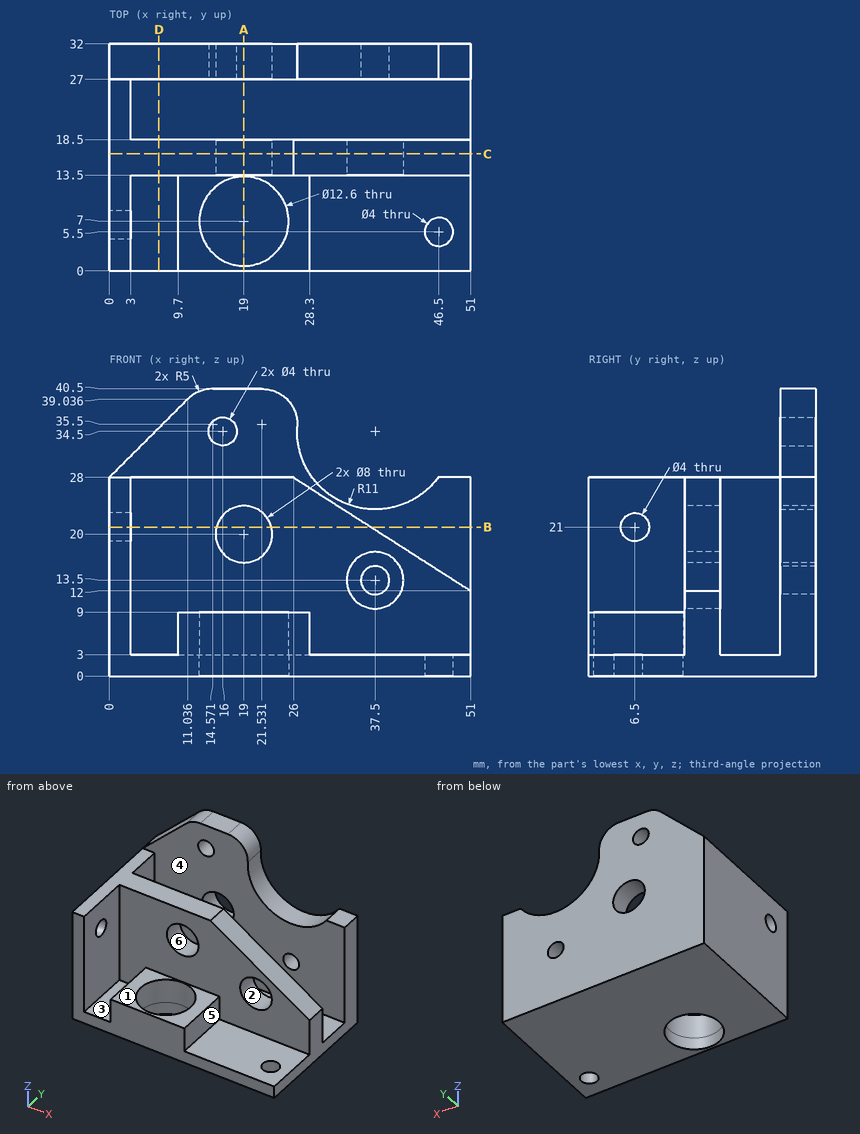
Part print with two shaded views. Sizes in mm from the minimum x, y, z corner. A direction names the side the tool comes from. Round coordinates to 2 decimals unless told otherwise and drop trailing zeros. Write each loop counter-clockwise with the first axis right and the second up, starting at its lowest first coordinate (ties: lowest second). Pieces come first, ordered by that corner, then holes. Notation, with made-up numbers: (-19.75, 60) - (28.25, 60) arc R34 ccw to (28.25, 90) - close; hole circle Ø7 at (-22.5, 8.25). An arc over 180 degrees is marked (long way). Use CSV: the item, a comma, the result in double quotes.
Item 1: Slice it at A-A, the plane x = 19. Write the cut outline in (y, z).
Results list:
outline,"(0, 0) - (0.7, 0) - (0.7, 9) - (0, 9) - close; (13.3, 0) - (32, 0) - (32, 16) - (27, 16) - (27, 3) - (18.5, 3) - (18.5, 16) - (13.5, 16) - (13.5, 9) - (13.3, 9) - close; (13.5, 24) - (18.5, 24) - (18.5, 28) - (13.5, 28) - close; (27, 24) - (32, 24) - (32, 40.5) - (27, 40.5) - close"
Item 2: Flat gauge pins, fed straight in: P1, Ø3.5, axis at y = 6.5, z = 21, coming from the -X side; P2, Ø4, axis at y = 22, z = 18, coming from the +X side; P3, Ø3, axis at x = 16.5, y = 21, coming from the +Z side; P4, Ø1.8, axis at y = 9, z = 5, coming from the +X side. Where does each tip first touch, or does it go through?
Results list:
P1,"passes through"
P2,"stops at x = 3"
P3,"stops at z = 3"
P4,"stops at x = 28.3"
Item 3: Slice it at B-B, the plane z = 21. Write the cut outline in (x, y), then the cut area to 3 significant figures.
Results list:
outline,"(0, 0) - (3, 0) - (3, 4.5) - (0, 4.5) - close; (0, 8.5) - (3, 8.5) - (3, 13.5) - (15.13, 13.5) - (15.13, 18.5) - (3, 18.5) - (3, 27) - (15.13, 27) - (15.13, 32) - (0, 32) - close; (22.87, 13.5) - (36.94, 13.5) - (36.94, 18.5) - (22.87, 18.5) - close; (22.87, 27) - (51, 27) - (51, 32) - (22.87, 32) - close"
area,"416 mm²"
Item 4: Slice it at D-D, the plane x = 7. Write the cut outline in (y, z).
Results list:
outline,"(0, 0) - (32, 0) - (32, 35) - (27, 35) - (27, 3) - (18.5, 3) - (18.5, 28) - (13.5, 28) - (13.5, 3) - (0, 3) - close"
Item 5: Pull direction X, two halves, no side cores. Call the marked faces 4, 5 and 6: pulls with the +X half, pulls with the -X half, needs draft (parallel to the pull), parting line crosses it, or undercut.
Results list:
face 4,"needs draft"
face 5,"pulls with the +X half"
face 6,"undercut"
Item 6: Slice it at C-C, the plane y = 16.5. Write the cut outline in (x, z).
Results list:
outline,"(0, 0) - (51, 0) - (51, 12) - (26, 28) - (0, 28) - close; hole circle Ø8 at (19, 20); hole circle Ø8 at (37.5, 13.5)"
Item 7: Tool access for the marked faces 1, 2 and 3: list every direction of +Z, -Z, +X, -X, +Y, -Y with a clear straight run to the whole face (end or side of a thin tool).
Results list:
face 1,"+Z, +X, -Y"
face 2,"-Y"
face 3,"+Z, -Y"
Item 8: Wall check: L1, parallel to Y at x = 33, z = 7; L2, parallel to Z at x = 19, y = 28; L3, parallel to X at y = 9.5, z = 5. Give the ranges that are in metal, low to high.
Results list:
L1,"y = 13.5 to 18.5, 27 to 32"
L2,"z = 0 to 16, 24 to 40.5"
L3,"x = 0 to 3, 9.7 to 13.22, 24.78 to 28.3"
